```python
from build123d import *

# Parameters (mm, degrees)
BOSS_EXTRUDE1_DEPTH = 6.6
SKETCH3_R           = 1
CUT_EXTRUDE1_DEPTH  = 6.6
BOSS_EXTRUDE2_DEPTH = 6.6
CHAMFER1_SIZE       = 0.4
FILLET1_R           = 0.4
FILLET2_R           = 0.4
RIB17_START         = -1.5
RIB17_DEPTH         = 3
SKETCH25_R          = 1
CUT_EXTRUDE2_DEPTH  = 13.2


# Read off the part's stored shape, not the designer's step: Rib17
with BuildPart() as part:
    # Sketch1 → Boss-Extrude1 (new, symmetric)
    with BuildSketch(Plane.XY):
        with BuildLine():
            Line((-0.5, 13.2), (-3.5, 13.2))
            Line((-3.5, 13.2), (-3.5, 9.367496998))
            ThreePointArc((-3.5, 9.367496998), (0, -10), (3.5, 9.367496998))
            Line((3.5, 9.367496998), (3.5, 13.2))
            Line((3.5, 13.2), (0.5, 13.2))
            Line((0.5, 13.2), (0.5, 6.982120022))
            ThreePointArc((0.5, 6.982120022), (5.123475383, 4.769696007), (7, 0))
            ThreePointArc((7, 0), (-4.769696007, -5.123475383), (-0.5, 6.982120022))
            Line((-0.5, 6.982120022), (-0.5, 13.2))
        make_face()
    extrude(amount=BOSS_EXTRUDE1_DEPTH, both=True)

    # Sketch3 → Cut-Extrude1 (cut, symmetric)
    with BuildSketch(Plane(origin=(0, 0, 0), x_dir=(0, 0, -1), z_dir=(1, 0, 0))):
        with Locations(Location((0, 11.283748499, 0), (0, 0, 180))):
            Circle(SKETCH3_R)
        with Locations(Location((4.001379793, 11.283748499, 0), (0, 0, 180))):
            Circle(SKETCH3_R)
        with Locations(Location((-4.00303992, 11.283748499, 0), (0, 0, 180))):
            Circle(SKETCH3_R)
    extrude(amount=CUT_EXTRUDE1_DEPTH, both=True, mode=Mode.SUBTRACT)

    # Sketch4 → Boss-Extrude2 (add, symmetric)
    with BuildSketch(Plane.XY):
        with BuildLine():
            Line((-10, 0), (-10, -12))
            Line((-10, -12), (-14, -12))
            Line((-14, -12), (-14, -16))
            Line((-14, -16), (-7, -16))
            Line((-7, -16), (-7, -7.141428429))
            ThreePointArc((-7, -7.141428429), (-9.219544457, -3.872983346), (-10, 0))
        make_face()
        with BuildLine():
            Line((10, 0), (10, -12))
            Line((10, -12), (14, -12))
            Line((14, -12), (14, -16))
            Line((14, -16), (7, -16))
            Line((7, -16), (7, -7.141428429))
            ThreePointArc((7, -7.141428429), (9.219544457, -3.872983346), (10, 0))
        make_face()
    extrude(amount=BOSS_EXTRUDE2_DEPTH, both=True)

    # Chamfer1
    chamfer1_edges = [part.edges().sort_by_distance(p)[0] for p in [
        (-7, -16, 0),
        (7, -16, 0),
    ]]
    chamfer(chamfer1_edges, length=CHAMFER1_SIZE)

    # Fillet1
    fillet1_edges = [part.edges().sort_by_distance(p)[0] for p in [
        (-10, -12, 0),
        (10, -12, 0),
    ]]
    fillet(fillet1_edges, radius=FILLET1_R)

    # Fillet2
    fillet2_edges = [part.edges().sort_by_distance(p)[0] for p in [
        (2, 13.2, -6.6),
        (-2, 13.2, -6.6),
        (-2, 13.2, 6.6),
        (2, 13.2, 6.6),
    ]]
    fillet(fillet2_edges, radius=FILLET2_R)

    # Rib17 outline → Rib17 (add)
    with BuildSketch(Plane.XY.offset(RIB17_START)):
        with BuildLine():
            Line((14, -12), (10, 0))
            Line((10, 0), (10, -11.6))
            ThreePointArc((10, -11.6), (10.117157288, -11.882842712), (10.4, -12))
            Line((10.4, -12), (14, -12))
        make_face()
    rib17 = extrude(amount=RIB17_DEPTH)

    # Mirror1: Rib17 across plane
    add(rib17.mirror(Plane(origin=(0, 0, 0), x_dir=(0, 0, 1), z_dir=(1, 0, 0))))

    # Sketch25 → Cut-Extrude2 (cut)
    with BuildSketch(Plane(origin=(0, -12, 0), x_dir=(1, 0, 0), z_dir=(0, 1, 0))):
        with Locations(Location((-12.2, 3.8, 0), (0, 0, 270))):
            Circle(SKETCH25_R)
        with Locations(Location((-12.2, -3.8, 0), (0, 0, 270))):
            Circle(SKETCH25_R)
        with Locations(Location((12.2, 3.8, 0), (0, 0, 270))):
            Circle(SKETCH25_R)
        with Locations(Location((12.2, -3.8, 0), (0, 0, 270))):
            Circle(SKETCH25_R)
    extrude(amount=-CUT_EXTRUDE2_DEPTH, mode=Mode.SUBTRACT)


solid = part.part
```
The listing builds one solid part. Answer for the finished solid, in the listing's coordinates (mm). A direction names the side the tool comes from. Coordinates: 2 decimals unless noted, no trailing zeros. Loops run counter-clockwise (first coordinate to the right, second up) from the corner with the lowest first, then second, coordinate; pieces in that order, holes last. Notation, with made-up numbers: M 89.5,12 L 121.5,12 A25 ccw 121.5,38 Z; hole C 74.25,67.25 d4. An arc over 180 degrees is marked long. Answer as a JSON object with one key per item and string values. Group by question number.
Item 1: Which of the six approach directions +Z, -Z, +X, -X, +Y, -Y give full straight-line access (tool end or side, diameter ignored) to faces 5 (the face through (-11, -9, 1.5)), 6 (the face through (-3.5, 13, 0)), 7 (the face through (11, -12, -5)), 8 (the face through (1.979, 10.292, -4.132)), 9 (the face through (-11, -9, -1.5))?
Item 2: Section C-C (y = -4.5) is taken. Write down the section's boundary in (x, z).
Item 3: Section D-D (x = -12.2) is taken. Write down the section's boundary in (y, z), and give its area (3 significant figures).
Item 4: Determine the mould class of faces 1 (the face through (10, -6, 4)), 2 (the face through (-10, -6, 4)), 3 (the face through (0.5, 10, 0)), 4 (the face through (2, 13.2, 0)) for opening direction X: +X half, -X half, draft (parallel to the pull), parting line (faces both ways), or undercut.
Item 5: Section B-B (x = 1) is taken. Write down the section's boundary in (y, z), and give its area (3 significant figures).
Item 6: Section A-A (y = -12.75) is taken. Write down the section's boundary in (x, z), and give its area (3 significant figures).
Item 7: Consider L1, parallel to X at y = -14.3, z = 3.8; L2, parallel to Y at x = 3.25, z = -3.25; L3, parallel to Z at x = 2.75, y = 11. Determine where each line is inside the solid, lowest interval first.
Item 8: Each of these flat-tipped pins is pushed along its axis until it touches: P1, Ø3, axis at x = 12.5, z = -4, coming from the +Y side; P2, Ø1.5, axis at y = -6.5, z = 0, coming from the +X side; P3, Ø4, axis at y = 12, z = -3, coming from the -X side. Where does it stop, or does it pass through?
Solved:
{
 "1": {"face 5": "+Z, -X, +Y", "face 6": "+Z, -Z, -X, +Y", "face 7": "-Z, +X, +Y", "face 8": "+X, -X", "face 9": "-Z, -X, +Y"},
 "2": {"outline": "M -11.5,-1.5 L -10,-1.5 L -10,-6.6 L -5.36,-6.6 L -5.36,6.6 L -10,6.6 L -10,1.5 L -11.5,1.5 Z; M 5.36,-6.6 L 10,-6.6 L 10,-1.5 L 11.5,-1.5 L 11.5,1.5 L 10,1.5 L 10,6.6 L 5.36,6.6 Z"},
 "3": {"outline": "M -16,-6.6 L -12,-6.6 L -12,-4.8 L -16,-4.8 Z; M -16,-2.8 L -12,-2.8 L -12,-1.5 L -6.6,-1.5 L -6.6,1.5 L -12,1.5 L -12,2.8 L -16,2.8 Z; M -16,4.8 L -12,4.8 L -12,6.6 L -16,6.6 Z", "area": "53.0 mm2"},
 "4": {"face 1": "+X half", "face 2": "-X half", "face 3": "undercut", "face 4": "draft"},
 "5": {"outline": "M -9.95,-6.6 L -6.93,-6.6 L -6.93,6.6 L -9.95,6.6 Z; M 6.93,-6.6 L 12.8,-6.6 A0.4 ccw 13.2,-6.2 L 13.2,6.2 A0.4 ccw 12.8,6.6 L 6.93,6.6 Z; hole C 11.28,-4 d2; hole C 11.28,0 d2; hole C 11.28,4 d2", "area": "113 mm2"},
 "6": {"outline": "M -14,-6.6 L -7,-6.6 L -7,6.6 L -14,6.6 Z; M 7,-6.6 L 14,-6.6 L 14,6.6 L 7,6.6 Z; hole C -12.2,-3.8 d2; hole C -12.2,3.8 d2; hole C 12.2,-3.8 d2; hole C 12.2,3.8 d2", "area": "172 mm2"},
 "7": {"L1": "x = -14 to -13.2, -11.2 to -7, 7 to 11.2, 13.2 to 14", "L2": "y = -9.46 to -6.2, 6.2 to 10.62, 11.94 to 13.2", "L3": "z = -6.6 to -4.96, -3.04 to -0.96, 0.96 to 3.04, 4.96 to 6.6"},
 "8": {"P1": "stops at y = -12", "P2": "stops at x = 12.42", "P3": "stops at x = -3.5"}
}
